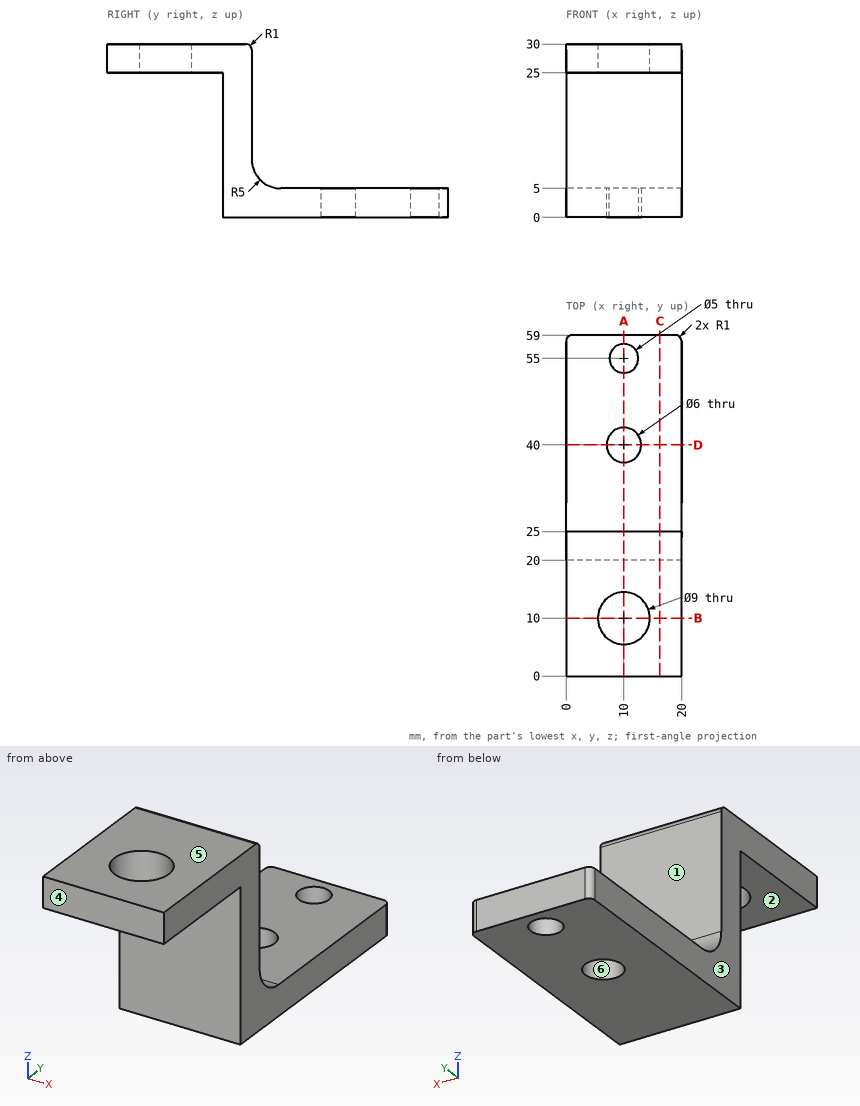
For this review, use the dimensioned drawing (mm, ordinates from the lowest corner) and the shaded views. A direction names the side the tool comes from. Round coordinates to 2 decimals unless told otherwise and drop trailing zeros. Loops run counter-clockwise (first coordinate to the right, second up) from the corner with the lowest first, then second, coordinate; pieces in that order, holes last. Notation, with made-up numbers: (-35, -31.75) -> (-15, -31.75) arc R27 cw to (-15, 2.25) -> close; hole circle Ø9 at (80, 21). An arc over 180 degrees is marked (long way). Write item = value, one per line. Start each with the question number.
Item 1: To check wall thickness, follow L1, parallel to Y at x = 10, z = 1.2; L2, parallel to Y at x = 10, z = 28.5; L3, parallel to Z at x = 14.25, y = 19. State the ranges of each line that lie inside material, in increasing order.
Item 2: Take a section at D-D on y = 40. Give the boundary of the cut face in (x, z).
Item 3: Take a section at B-B on y = 10. Give the boundary of the cut face in (x, z), plus the area to 3 significant figures.
Item 4: For the marked faces 1, 2 and 3, list the 3-axis set-ups (+Z, -Z, +X, -X, +Y, -Y) from which the entire face can be reached by the end or side of a thin tool; tool diameter is ignored.
Item 5: Take a section at C-C on x = 16.25. Give the boundary of the cut face in (y, z).
Item 6: Insertion check: pin 1 (12 mm diameter, centred on y = 47.5, z = 13, fed in from +X); pin 2 (12 mm diameter, centred on x = 6.5, y = 33, fed in from -Z); pin 3 (6 mm diameter, centred on x = 10, y = 55, fed in from +Z); pin 4 (11.5 mm diameter, centred on x = 10, y = 10, fed in from -Z). Each pin has a flat end and moves straight along its axis. Give the tip position at first contact, or say it passes through.
Item 7: Mouldability with a two-part tool opening along Y and no side actions: class the marked faces 4, 5 and 6 as released by +Y, released by -Y, zero draft, split by the parting line, or undercut.
Item 8: Take a section at A-A on x = 10. Give the boundary of the cut face in (y, z), plus the area to 3 significant figures.
Result:
q1.L1 = 20 to 37, 43 to 52.5, 57.5 to 59
q1.L2 = 0 to 5.5, 14.5 to 25
q1.L3 = 25 to 30
q2.outline = (0, 0) -> (7, 0) -> (7, 5) -> (0, 5) -> close; (13, 0) -> (20, 0) -> (20, 5) -> (13, 5) -> close
q3.outline = (0, 25) -> (5.5, 25) -> (5.5, 30) -> (0, 30) -> close; (14.5, 25) -> (20, 25) -> (20, 30) -> (14.5, 30) -> close
q3.area = 55.0 mm²
q4.face_1 = +Z, +X, -X, +Y
q4.face_2 = -Z, +X, -X, -Y
q4.face_3 = +Z, -Z, -X, +Y, -Y
q5.outline = (0, 25) -> (20, 25) -> (20, 0) -> (59, 0) -> (59, 5) -> (30, 5) arc R5 cw to (25, 10) -> (25, 29) arc R1 ccw to (24, 30) -> (0, 30) -> close
q6.pin_1 = through
q6.pin_2 = 0
q6.pin_3 = 5
q6.pin_4 = 25
q7.face_4 = released by -Y
q7.face_5 = zero draft
q7.face_6 = undercut
q8.outline = (0, 25) -> (5.5, 25) -> (5.5, 30) -> (0, 30) -> close; (14.5, 25) -> (20, 25) -> (20, 0) -> (37, 0) -> (37, 5) -> (30, 5) arc R5 cw to (25, 10) -> (25, 29) arc R1 ccw to (24, 30) -> (14.5, 30) -> close; (43, 0) -> (52.5, 0) -> (52.5, 5) -> (43, 5) -> close; (57.5, 0) -> (59, 0) -> (59, 5) -> (57.5, 5) -> close
q8.area = 325 mm²
